Build history of the part. All positions in model axes, mm. A direction names the side the tool comes from. Give positions to 0.01 mm unless a question says otherwise; leave off trailing zeros. Order: outer loops, then holes, each group sorted by start corner. A loop starts at its lowest first (then second) coordinate and runs counter-clockwise, first axis right, second up. Notation, with made-up numbers: (-23.75, -11) -> (0.25, -11) arc R7 ccw to (0.25, -5) -> close; hole circle Ø3 at (-2, -15). An arc over 180 degrees is marked (long way). One line per question, with ' | ' between items. Start each with the question number.
(1) Drill centre lines: L1, parallel to Y at x = -16, z = 28; L2, parallel to Z at x = 1.5, y = 13; L3, parallel to Z at x = 5.5, y = 25.5. Where is each one in solid material? Low to high. Write a range as from..to.
(2) Pin check, flat tips, straight feed: pin 1 Ø5 at (x, y) = (10, -10) entering from +Z; pin 2 Ø5 at (x, y) = (16.5, 46) entering from -Z; pin 3 Ø5 at (x, z) = (1.5, 6) entering from +Y; pin 4 Ø1.8 at (x, y) = (-10, 10) entering from +Z. Stop position of each tip, or through.
(3) Pull direction Y, two halves, no side cores. Call faces 4 (the face through (-0.388, -17.177, -1.22)), 5 (the face through (-24.667, -16.986, 28.737)), 6 (the face through (8.8, -10.9, -1)): +Y half, -Y half, draft (parallel to the pull), parting line (faces both ways), or undercut.
(4) Cut at A-A (z = 17.5). Give the cut face in (x, y).
(5) Cut at D-D (x = -10). Give the cut face in (y, z).
(6) Cut at C-C (y = -10). Give the cut face in (x, z).
(7) Which spindle directions (+Z, -Z, +X, -X, +Y, -Y) get a long thin tool onto all of the face, cutting with end or side? Do faces 1 (the face through (0, 18, 20)), 2 (the face through (24.667, -16.986, 28.737)), 3 (the face through (0, 0, 0)). Say none if no direction does.
(8) Cut at B-B (x = 24.7). Give the number of separate pieces and of enclosed holes in the cut face, then the cut area to 3 significant figures.
from build123d import *

# Parameters (mm, degrees)
SZKIC1_W                             = 55.4
SZKIC1_H                             = 32
ODGI_CIE_BAZOWE1_DEPTH               = 2
OTWORY_USTALAJ_CE_3_0MM1_D           = 3
OTWORY_USTALAJ_CE_3_0MM1_DEPTH       = 17
OTWORY_USTALAJ_CE_3_0MM1_TIP         = 0.901290929
ODGI_CIE_KRAW_DZI1_STRIP_W           = 9.4732
ODGI_CIE_KRAW_DZI1_STRIP_H           = 2
ODGI_CIE_KRAW_DZI1_STRIP_CUT_DEPTH   = 55.4
ODGI_CIE_KRAW_DZI1_STRIP_2_W         = 9.4732
ODGI_CIE_KRAW_DZI1_STRIP_2_H         = 2
ODGI_CIE_KRAW_DZI1_STRIP_CUT_2_DEPTH = 55.4
ODGI_CIE_KRAW_DZI1_DEPTH             = 55.4
ODGI_CIE_KRAW_DZI1_BEND_DEPTH        = 55.4
ODGI_CIE_KRAW_DZI2_STRIP_W           = 9.4732
ODGI_CIE_KRAW_DZI2_STRIP_H           = 2
ODGI_CIE_KRAW_DZI2_STRIP_CUT_DEPTH   = 55.4
ODGI_CIE_KRAW_DZI2_DEPTH             = 55.4
WYTNIJ_WYCI_GNI_CIE1_DEPTH           = 66.53846199


# Sheet-metal steps are written as plain solids
with BuildPart() as part:
    # Szkic1 → Odgięcie bazowe1 (new body)
    with BuildSketch(Plane.XY):
        Rectangle(SZKIC1_W, SZKIC1_H)
    extrude(amount=-ODGI_CIE_BAZOWE1_DEPTH)

    # Otwory ustalające Ø3.0mm1
    with Locations(Plane(origin=(0, 0, -2), x_dir=(-1, 0, 0), z_dir=(0, 0, -1))):
        with Locations((-10, 10), (10, 10), (10, -10), (-10, -10)):
            Hole(OTWORY_USTALAJ_CE_3_0MM1_D / 2, depth=OTWORY_USTALAJ_CE_3_0MM1_DEPTH)
            with Locations((0, 0, -(OTWORY_USTALAJ_CE_3_0MM1_DEPTH + OTWORY_USTALAJ_CE_3_0MM1_TIP / 2))):  # 118° drill point
                Cone(0, OTWORY_USTALAJ_CE_3_0MM1_D / 2, OTWORY_USTALAJ_CE_3_0MM1_TIP, mode=Mode.SUBTRACT)

    # Odgięcie krawędzi1 strip (across the edge) → Odgięcie krawędzi1 strip cut (cut)
    with BuildSketch(Plane(origin=(27.7, 16, 0), x_dir=(0, -1, 0), z_dir=(-1, 0, 0))):
        with Locations((-4, -1)):
            Rectangle(ODGI_CIE_KRAW_DZI1_STRIP_W, ODGI_CIE_KRAW_DZI1_STRIP_H)
    extrude(amount=ODGI_CIE_KRAW_DZI1_STRIP_CUT_DEPTH, mode=Mode.SUBTRACT)

    # Odgięcie krawędzi1 strip 2 (across the edge) → Odgięcie krawędzi1 strip cut 2 (cut)
    with BuildSketch(Plane(origin=(-27.7, -16, 0), x_dir=(0, 1, 0), z_dir=(1, 0, 0))):
        with Locations((-4, -1)):
            Rectangle(ODGI_CIE_KRAW_DZI1_STRIP_2_W, ODGI_CIE_KRAW_DZI1_STRIP_2_H)
    extrude(amount=ODGI_CIE_KRAW_DZI1_STRIP_CUT_2_DEPTH, mode=Mode.SUBTRACT)

    # Odgięcie krawędzi1 section (across the edge) → Odgięcie krawędzi1 (add)
    with BuildSketch(Plane(origin=(27.7, 16, 0), x_dir=(0, -1, 0), z_dir=(-1, 0, 0))):
        with BuildLine():
            Line((-2, 0.7366), (-2, 40))
            Line((-2, 40), (0, 40))
            Line((0, 40), (0, 0.7366))
            ThreePointArc((0, 0.7366), (0.215745145, 0.215745145), (0.7366, 0))
            Line((0.7366, 0), (0.7366, -2))
            ThreePointArc((0.7366, -2), (-1.198468417, -1.198468417), (-2, 0.7366))
        make_face()
    extrude(amount=ODGI_CIE_KRAW_DZI1_DEPTH)

    # Odgięcie krawędzi1 section 2 (across the edge) → Odgięcie krawędzi1 bend (add)
    with BuildSketch(Plane(origin=(-27.7, -16, 0), x_dir=(0, 1, 0), z_dir=(1, 0, 0))):
        with BuildLine():
            Line((-2, 0.7366), (-2, 40))
            Line((-2, 40), (0, 40))
            Line((0, 40), (0, 0.7366))
            ThreePointArc((0, 0.7366), (0.215745145, 0.215745145), (0.7366, 0))
            Line((0.7366, 0), (0.7366, -2))
            ThreePointArc((0.7366, -2), (-1.198468417, -1.198468417), (-2, 0.7366))
        make_face()
    extrude(amount=ODGI_CIE_KRAW_DZI1_BEND_DEPTH)

    # Odgięcie krawędzi2 strip (across the edge) → Odgięcie krawędzi2 strip cut (cut)
    with BuildSketch(Plane(origin=(-27.7, 18, 40), x_dir=(0, 0, -1), z_dir=(1, 0, 0))):
        with Locations((-4, -1)):
            Rectangle(ODGI_CIE_KRAW_DZI2_STRIP_W, ODGI_CIE_KRAW_DZI2_STRIP_H)
    extrude(amount=ODGI_CIE_KRAW_DZI2_STRIP_CUT_DEPTH, mode=Mode.SUBTRACT)

    # Odgięcie krawędzi2 section (across the edge) → Odgięcie krawędzi2 (add)
    with BuildSketch(Plane(origin=(-27.7, 18, 40), x_dir=(0, 0, -1), z_dir=(1, 0, 0))):
        with BuildLine():
            Line((-2, 0.7366), (-2, 42))
            Line((-2, 42), (0, 42))
            Line((0, 42), (0, 0.7366))
            ThreePointArc((0, 0.7366), (0.215745145, 0.215745145), (0.7366, 0))
            Line((0.7366, 0), (0.7366, -2))
            ThreePointArc((0.7366, -2), (-1.198468417, -1.198468417), (-2, 0.7366))
        make_face()
    extrude(amount=ODGI_CIE_KRAW_DZI2_DEPTH)

    # Szkic16 → Wytnij-wyciągnięcie1 (cut, through all)
    with BuildSketch(Plane(origin=(0, 18, 0), x_dir=(1, 0, 0), z_dir=(0, 1, 0))):
        with BuildLine():
            Line((26.2, -30.2366), (26.2, -31.2366))
            ThreePointArc((26.2, -31.2366), (24.7, -32.7366), (23.2, -31.2366))
            Line((23.2, -31.2366), (23.2, -30.2366))
            ThreePointArc((23.2, -30.2366), (24.7, -28.7366), (26.2, -30.2366))
        make_face()
        with BuildLine():
            Line((26.2, -10.2366), (26.2, -11.2366))
            ThreePointArc((26.2, -11.2366), (24.7, -12.7366), (23.2, -11.2366))
            Line((23.2, -11.2366), (23.2, -10.2366))
            ThreePointArc((23.2, -10.2366), (24.7, -8.7366), (26.2, -10.2366))
        make_face()
        with BuildLine():
            Line((-26.2, -10.2366), (-26.2, -11.2366))
            ThreePointArc((-26.2, -11.2366), (-24.7, -12.7366), (-23.2, -11.2366))
            Line((-23.2, -11.2366), (-23.2, -10.2366))
            ThreePointArc((-23.2, -10.2366), (-24.7, -8.7366), (-26.2, -10.2366))
        make_face()
        with BuildLine():
            Line((-26.2, -30.2366), (-26.2, -31.2366))
            ThreePointArc((-26.2, -31.2366), (-24.7, -32.7366), (-23.2, -31.2366))
            Line((-23.2, -31.2366), (-23.2, -30.2366))
            ThreePointArc((-23.2, -30.2366), (-24.7, -28.7366), (-26.2, -30.2366))
        make_face()
    extrude(amount=-WYTNIJ_WYCI_GNI_CIE1_DEPTH, mode=Mode.SUBTRACT)


solid = part.part
Result set:
1) L1: y = -18..-16, 16..18 | L2: z = -2..0 | L3: z = 40..42
2) pin 1: stops at z = 0 | pin 2: stops at z = 40 | pin 3: stops at y = 18 | pin 4: passes through
3) face 4: -Y half | face 5: draft | face 6: undercut
4) outline: (-27.7, -18) -> (27.7, -18) -> (27.7, -16) -> (-27.7, -16) -> close; (-27.7, 16) -> (27.7, 16) -> (27.7, 18) -> (-27.7, 18) -> close
5) outline: (-18, 0.74) arc R2.74 ccw to (-15.26, -2) -> (-11.5, -2) -> (-11.5, 0) -> (-15.26, 0) arc R0.74 cw to (-16, 0.74) -> (-16, 40) -> (-18, 40) -> close; (-8.5, -2) -> (8.5, -2) -> (8.5, 0) -> (-8.5, 0) -> close; (11.5, -2) -> (15.26, -2) arc R2.74 ccw to (18, 0.74) -> (18, 39.26) arc R0.74 cw to (18.74, 40) -> (60, 40) -> (60, 42) -> (18.74, 42) arc R2.74 ccw to (16, 39.26) -> (16, 0.74) arc R0.74 cw to (15.26, 0) -> (11.5, 0) -> close
6) outline: (-27.7, -2) -> (-11.5, -2) -> (-11.5, 0) -> (-27.7, 0) -> close; (-8.5, -2) -> (8.5, -2) -> (8.5, 0) -> (-8.5, 0) -> close; (11.5, -2) -> (27.7, -2) -> (27.7, 0) -> (11.5, 0) -> close
7) face 1: -Z, +X, -X, +Y | face 2: +Y, -Y | face 3: +Z, +X, -X
8) separate pieces: 5 | enclosed holes: 0 | area: 284 mm2
